Check sheet for the drawn part. Datum: minimum x, y, z corner. Units: mm. A direction names the side the tool comes from. Round coordinates to 2 decimals unless told otherwise and drop trailing zeros. Order: outer loops, then holes, each group sorted by start corner. A loop starts at its lowest first (then second) coordinate and runs counter-clockwise, first axis right, second up.
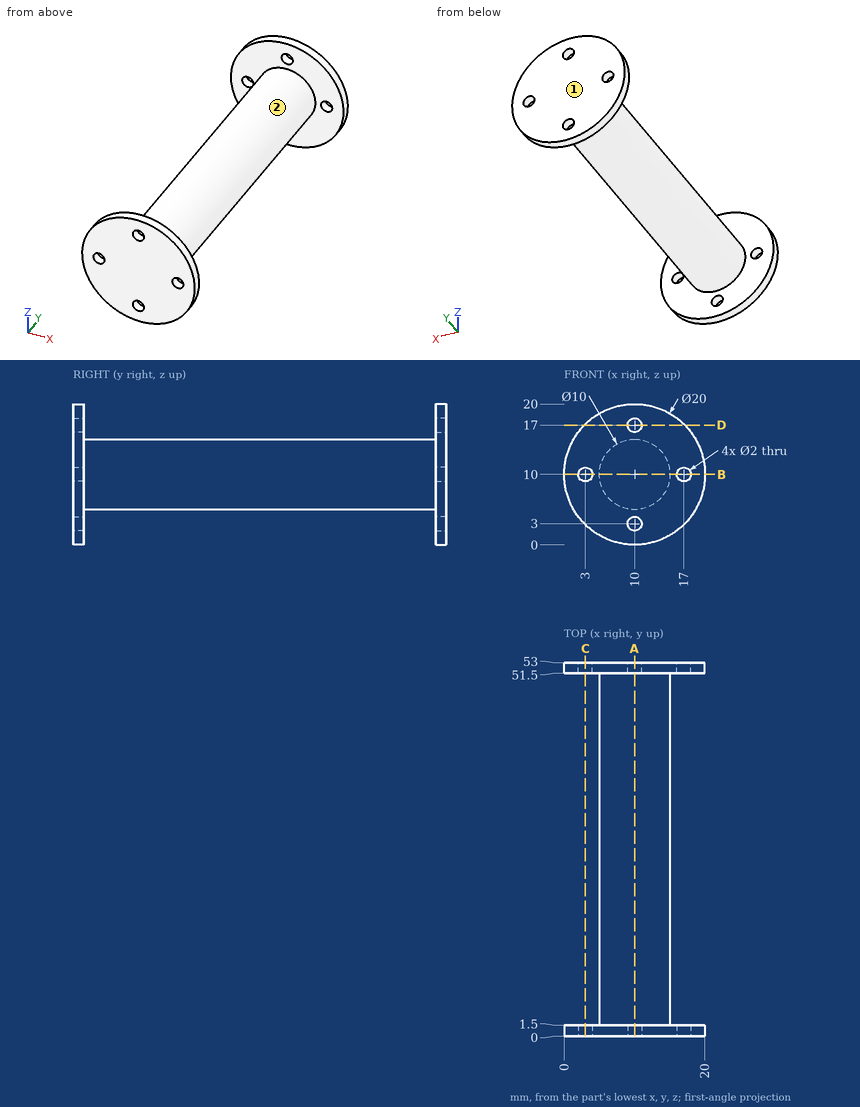
(1) Material ranges on line 1 (X direction, y = 52.3, z = 10); line 2 (Y direction, x = 14, z = 17.5); line 3 (X direction, y = 0.45, z = 3), recorded low to high.
Returned:
line 1: x = 0 to 2, 4 to 16, 18 to 20
line 2: y = 0 to 1.5, 51.5 to 53
line 3: x = 2.86 to 9, 11 to 17.14
(2) Sectioned sample at B-B, the plane z = 10. Record the cut outline in (x, y), and give its area (3 significant figures).
Returned:
outline: (0, 0) - (2, 0) - (2, 1.5) - (0, 1.5) - close; (0, 51.5) - (2, 51.5) - (2, 53) - (0, 53) - close; (4, 0) - (16, 0) - (16, 1.5) - (15, 1.5) - (15, 51.5) - (16, 51.5) - (16, 53) - (4, 53) - (4, 51.5) - (5, 51.5) - (5, 1.5) - (4, 1.5) - close; (18, 0) - (20, 0) - (20, 1.5) - (18, 1.5) - close; (18, 51.5) - (20, 51.5) - (20, 53) - (18, 53) - close
area: 548 mm2
(3) Sectioned sample at C-C, the plane x = 3. Record the cut outline in (y, z).
Returned:
outline: (0, 2.86) - (1.5, 2.86) - (1.5, 9) - (0, 9) - close; (0, 11) - (1.5, 11) - (1.5, 17.14) - (0, 17.14) - close; (51.5, 2.86) - (53, 2.86) - (53, 9) - (51.5, 9) - close; (51.5, 11) - (53, 11) - (53, 17.14) - (51.5, 17.14) - close
(4) Sectioned sample at A-A, the plane x = 10. Record the cut outline in (y, z), and give its area (3 significant figures).
Returned:
outline: (0, 0) - (1.5, 0) - (1.5, 2) - (0, 2) - close; (0, 4) - (1.5, 4) - (1.5, 5) - (51.5, 5) - (51.5, 4) - (53, 4) - (53, 16) - (51.5, 16) - (51.5, 15) - (1.5, 15) - (1.5, 16) - (0, 16) - close; (0, 18) - (1.5, 18) - (1.5, 20) - (0, 20) - close; (51.5, 0) - (53, 0) - (53, 2) - (51.5, 2) - close; (51.5, 18) - (53, 18) - (53, 20) - (51.5, 20) - close
area: 548 mm2
(5) Depth check by flat-ended pin: P1, Ø2.5, axis at x = 3, z = 10, coming from the +Y side; P2, Ø6, axis at x = 10.5, y = 42.5, coming from the -Z side; P3, Ø1.6, axis at x = 10, z = 3, coming from the +Y side; P4, Ø6, axis at x = 10.5, y = 44.5, coming from the +Z side. Enter the tip coordinate at first touch or a pass-through.
Returned:
P1: stops at y = 53
P2: stops at z = 5
P3: passes through
P4: stops at z = 15
(6) Sectioned sample at D-D, the plane z = 17. Record the cut outline in (x, y), and give its area (3 significant figures).
Returned:
outline: (2.86, 0) - (9, 0) - (9, 1.5) - (2.86, 1.5) - close; (2.86, 51.5) - (9, 51.5) - (9, 53) - (2.86, 53) - close; (11, 0) - (17.14, 0) - (17.14, 1.5) - (11, 1.5) - close; (11, 51.5) - (17.14, 51.5) - (17.14, 53) - (11, 53) - close
area: 36.8 mm2
(7) Set-up check for the marked faces 1 and 2: record each of +Z, -Z, +X, -X, +Y, -Y from which the full face is reachable in a straight line by a thin tool's end or side.
Returned:
face 1: +Z, -Z, +X, -X, +Y
face 2: none
